Read the model definition and answer for the solid it produces. Units are mm, in the model's axes. Face numbers are marked on the shaded views. A direction names the side the tool comes from. Coordinates: 2 decimals unless noted, no trailing zeros. Order: outer loops, then holes, each group sorted by start corner. A loop starts at its lowest first (then second) coordinate and runs counter-clockwise, first axis right, second up. Notation, with made-up numbers: (72.5, 83.25) - (87.5, 83.25) arc R23 ccw to (87.5, 95.25) - close; hole circle Ø3 at (-9, 6). An arc over 180 degrees is marked (long way). Use one line per item in the form item = value.
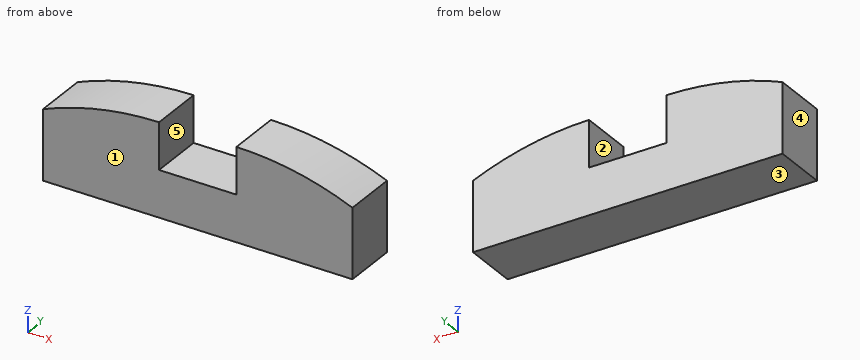
```python
from build123d import *

# Parameters (mm, degrees)
F0_W     = 38.1
F0_H     = 17.78
F0_W_2   = 25.4
F1_DEPTH = 15.24
F2_DEPTH = 15.24
F4_DEPTH = 25.4


with BuildPart() as f1:
    # F0 (on Top) → F1 (new body)
    with BuildSketch(Plane.XY):
        with Locations((-19.05, -38.952387)):
            Rectangle(F0_W, F0_H)
        with Locations((12.7, -38.952387)):
            Rectangle(F0_W_2, F0_H)
        with Locations((44.45, -38.952387)):
            Rectangle(F0_W, F0_H)
    extrude(amount=-F1_DEPTH)

    # F0 (on Top) → F2 (join)
    with BuildSketch(Plane.XY):
        with Locations((-19.05, -38.952387)):
            Rectangle(F0_W, F0_H)
        with Locations((44.45, -38.952387)):
            Rectangle(F0_W, F0_H)
    extrude(amount=F2_DEPTH)

    # F3 (on face) → F4 (cut)
    with BuildSketch(Plane.XZ.offset(47.842387)):
        with BuildLine():
            ThreePointArc((-38.1, 7.62), (-19.427264, 13.316322), (0, 15.24))
            Line((0, 15.24), (-38.1, 15.24))
            Line((-38.1, 15.24), (-38.1, 7.62))
        make_face()
        with BuildLine():
            Line((63.5, 15.24), (25.4, 15.24))
            ThreePointArc((25.4, 15.24), (44.827264, 13.316322), (63.5, 7.62))
            Line((63.5, 7.62), (63.5, 15.24))
        make_face()
    extrude(amount=-F4_DEPTH, mode=Mode.SUBTRACT)


solid = f1.part
```
(1) The mould has two halves that part along X. Classify the marked faces 3, 4 and 5: +X half, -X half, draft (parallel to the pull), parting line (faces both ways), or undercut.
Answer list:
face_3 = draft
face_4 = -X half
face_5 = undercut
(2) Straight lines are drawn through the part: L1, parallel to X at y = -41, z = 1; L2, parallel to Z at x = 24.5, y = -40.25; L3, parallel to Z at x = -1, y = -31.75. For each, find the intervals that lie inside material, in ascending order.
Answer list:
L1 = -38.1 to 0, 25.4 to 63.5
L2 = -15.24 to 0
L3 = -15.24 to 15.23
(3) Given pin 1 Ø9 at (x, y) = (8.5, -37.5) entering from +Z; pin 2 Ø7.5 at (y, z) = (-38.5, 11) entering from -X; pin 3 Ø8 at (x, y) = (-11, -36) entering from +Z; pin 4 Ø5 at (y, z) = (-46, 10.5) entering from +X, each flat-ended and moving along its own axis, determine where each tip first touches the part or whether it passes through.
Answer list:
pin_1 = 0
pin_2 = -38.1
pin_3 = 14.99
pin_4 = 62.57
(4) Which of the six approach directions +Z, -Z, +X, -X, +Y, -Y give full straight-line access (tool end or side, diameter ignored) to the marked faces 1 and 2?
Answer list:
face_1 = +Z, -Z, +X, -X, -Y
face_2 = +Z, +Y, -Y
(5) Section B-B, the plane z = 8.5 is taken. Write down the section's boundary in (x, y), then the cut area to 3 significant figures.
Answer list:
outline = (-35.92, -47.84) - (0, -47.84) - (0, -30.06) - (-35.92, -30.06) - close; (25.4, -47.84) - (61.32, -47.84) - (61.32, -30.06) - (25.4, -30.06) - close
area = 1,280 mm2
(6) Section D-D, the plane x = -12.5 is taken. Write down the section's boundary in (y, z).
Answer list:
outline = (-47.84, -15.24) - (-30.06, -15.24) - (-30.06, 14.45) - (-47.84, 14.45) - close
(7) Section C-C, the plane x = 56.5 is taken. Write down the section's boundary in (y, z).
Answer list:
outline = (-47.84, -15.24) - (-30.06, -15.24) - (-30.06, 10.23) - (-47.84, 10.23) - close
(8) Section A-A, the plane y = -45.75 is taken. Write down the section's boundary in (x, z), then the cut area to 3 significant figures.
Answer list:
outline = (-38.1, -15.24) - (63.5, -15.24) - (63.5, 7.62) arc R99.06 ccw to (25.4, 15.24) - (25.4, 0) - (0, 0) - (0, 15.24) arc R99.06 ccw to (-38.1, 7.62) - close
area = 2,520 mm2
